Here's the drawing with two shaded views (mm, measured from the low corner). I have some questions. Coordinates: 2 decimals unless noted, no trailing zeros. Order: outer loops, then holes, each group sorted by start corner. A loop starts at its lowest first (then second) coordinate and runs counter-clockwise, first axis right, second up. Notation, with made-up numbers: (5.25, -30.5) -> (16.25, -30.5) arc R15 cw to (16.25, -14.5) -> close; hole circle Ø1 at (77.5, -4.75). An arc over 180 degrees is marked (long way). Write item = value, one per line.
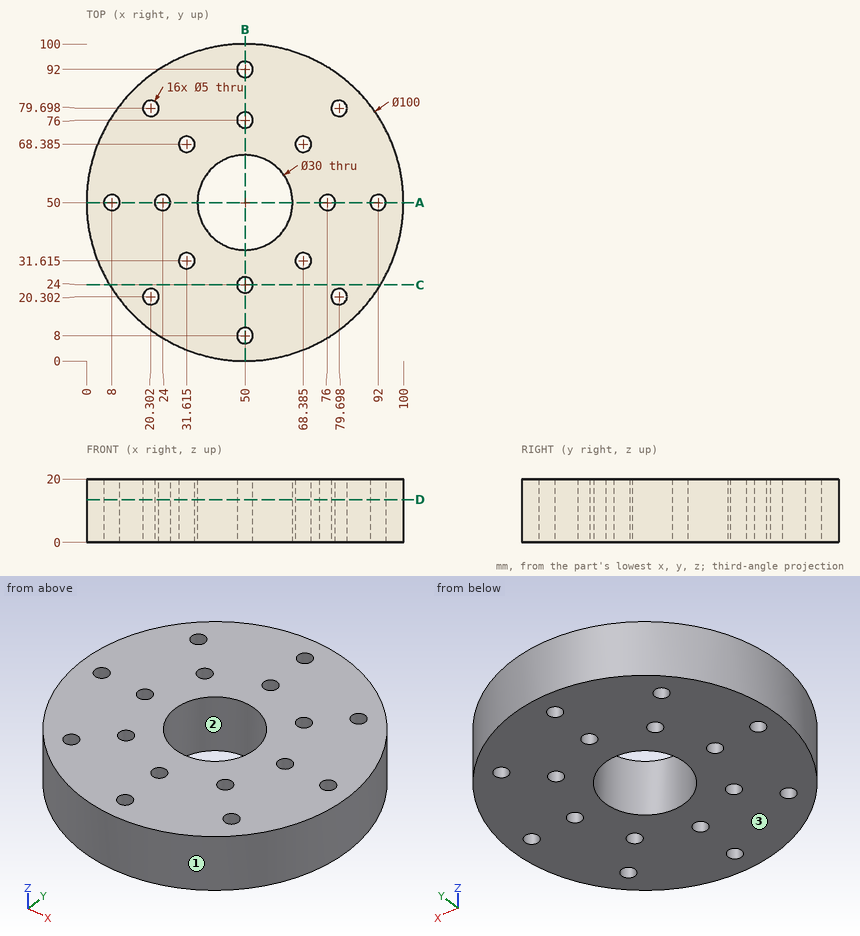
Item 1: I'm going to push flat-ended pins straight in: P1, Ø3, axis at y = 59.5, z = 17, coming from the +X side; P2, Ø1, axis at x = 74, z = 10.5, coming from the -Y side; P3, Ø1, axis at y = 36.5, z = 16, coming from the +X side. Where does each tip first touch, or does it pass through?
A:
P1 = 99.36
P2 = 5.87
P3 = 98.28
Item 2: If we mould it in two halves opening along Y, with no side actions, what happens to the marked faces 1, 2 and 3? For each: pulls with the +Y half, pulls with the -Y half, needs draft (parallel to the pull), parting line crosses it, or undercut.
A:
face_1 = parting line crosses it
face_2 = undercut
face_3 = needs draft
Item 3: If I drill on probe 1 along Y at (x, z) = (50, 11); probe 2 along X at (y, z) = (31.5, 16); probe 3 along Y at (x, z) = (32, 15.75) (1 decimal), over which ranges is the centre line in solid material (lowest first)?
A:
probe_1 = 0 to 5.5, 10.5 to 21.5, 26.5 to 35, 65 to 73.5, 78.5 to 89.5, 94.5 to 100
probe_2 = 3.55 to 29.12, 34.11 to 65.89, 70.88 to 96.45
probe_3 = 3.4 to 29.1, 34.1 to 65.9, 70.9 to 96.6
Item 4: I want a section at A-A, the plane y = 50. Please give me the cut outline in (x, z), plus the area to 3 significant figures.
A:
outline = (0, 0) -> (5.5, 0) -> (5.5, 20) -> (0, 20) -> close; (10.5, 0) -> (21.5, 0) -> (21.5, 20) -> (10.5, 20) -> close; (26.5, 0) -> (35, 0) -> (35, 20) -> (26.5, 20) -> close; (65, 0) -> (73.5, 0) -> (73.5, 20) -> (65, 20) -> close; (78.5, 0) -> (89.5, 0) -> (89.5, 20) -> (78.5, 20) -> close; (94.5, 0) -> (100, 0) -> (100, 20) -> (94.5, 20) -> close
area = 1,000 mm2
Item 5: I want a section at C-C, the plane y = 24. Please give me the cut outline in (x, z).
A:
outline = (7.29, 0) -> (47.5, 0) -> (47.5, 20) -> (7.29, 20) -> close; (52.5, 0) -> (92.71, 0) -> (92.71, 20) -> (52.5, 20) -> close
Item 6: I want a section at D-D, the plane z = 13.5. Give the number of separate pieces and of enclosed holes in the cut face, plus the area to 3 significant figures.
A:
separate_pieces = 1
enclosed_holes = 17
area = 6,830 mm2
